Can you work these out from the model? Positions are in its coordinate system, mm. A direction names the side the tool comes from. Round coordinates to 2 decimals unless told otherwise and drop trailing zeros. Order: outer loops, then holes, each group sorted by start corner. A loop starts at its lowest first (then second) coordinate and runs counter-clockwise, first axis right, second up. Notation, with made-up numbers: (-1, -25.5) -> (56, -25.5) arc R20 ccw to (56, 1.5) -> close; hole circle Ø8 at (80, 74.5). An arc over 180 degrees is marked (long way). Use a Markdown table: item, result. Add a question column.
Q1. For faces 5 (the face through (-104.944, -2.465, 3.44)), 6 (the face through (-2.5, -2, -60)), which set-ups out of +Z, -Z, +X, -X, +Y, -Y let a thin tool reach every point of the face, with its end or its side?
Q2. I'm going to push flat-ended pins straight in: pin 1 Ø1.5 at (y, z) = (-3.5, -79.5) entering from -X; pin 2 Ø2 at (x, y) = (-24, -3) entering from -Z; pin 3 Ø3 at (x, y) = (-54.5, -3.5) entering from -Z. Where does each tip first touch, or does it pass through?
Q3. We'd pull the mould along Z, two halves only. Please class faces 1 (the face through (-9.91, -2.46, -93.98)), 2 (the face through (83.17, -2.46, -44.87)), 3 (the face through (86.34, -2.46, 38.41)), 4 (the face through (2.5, -2, -64)): +Z half, -Z half, draft (parallel to the pull), parting line (faces both ways), or undercut.
Q4. I need wall thicknesses on line 1 along X through (y, z) = (-0.45, 17.5); line 2 along Z through (x, y) = (-35, -4.15); line 3 along Z through (x, y) = (-22.5, -3.2). Which ranges of each line are inside material? Lowest first, please. Write a range as [from, to].
Q5. If we section it at B-B on x = 74: List the corners of the cut face in (y, z) for me.
Q6. If we section it at A-A on z = 80: List the corners of the cut face in (x, y) for me, plus the area to 3 significant figures.
Q7. If we section it at C-C on x = -33: List the corners of the cut face in (y, z) for me, plus the area to 3 significant figures.
Q8. If we section it at D-D on x = -69.5: List the corners of the cut face in (y, z) for me.
```python
from build123d import *

# Parameters (mm, degrees)
EXTRUDE_1_DEPTH = 5
EXTRUDE_2_DEPTH = 5
FILLET_1_R      = 2


with BuildPart() as part:
    # 草圖1 → 填料-伸長1 (new body)
    with BuildSketch(Plane(origin=(0, 0, 0), x_dir=(1, 0, 0), z_dir=(0, 1, 0))):
        with BuildLine():
            Line((50.565945697, -26.307511014), (22.900635095, -10.334936491))
            Line((22.900635095, -10.334936491), (20.400635095, -14.665063509))
            Line((20.400635095, -14.665063509), (48.065945697, -30.637638033))
            ThreePointArc((48.065945697, -30.637638033), (30.4, -48.216594654), (6.922542226, -56.578073572))
            Line((6.922542226, -56.578073572), (4.437329437, -24.729741355))
            Line((4.437329437, -24.729741355), (-0.547516958, -25.118722602))
            Line((-0.547516958, -25.118722602), (1.93769583, -56.96705482))
            ThreePointArc((1.93769583, -56.96705482), (-26.556795854, -50.435469602), (-48.065945697, -30.637638033))
            Line((-48.065945697, -30.637638033), (-20.400635095, -14.665063509))
            Line((-20.400635095, -14.665063509), (-22.900635095, -10.334936491))
            Line((-22.900635095, -10.334936491), (-50.565945697, -26.307511014))
            ThreePointArc((-50.565945697, -26.307511014), (-56.956795854, -2.218874948), (-52.459320124, 22.29393936))
            Line((-52.459320124, 22.29393936), (-23.635248961, 8.522030659))
            Line((-23.635248961, 8.522030659), (-21.479693405, 13.033524896))
            Line((-21.479693405, 13.033524896), (-50.303764568, 26.805433596))
            ThreePointArc((-50.303764568, 26.805433596), (-30.4, 48.216594654), (-2.5, 56.945149047))
            Line((-2.5, 56.945149047), (-2.5, 25))
            Line((-2.5, 25), (2.5, 25))
            Line((2.5, 25), (2.5, 56.945149047))
            ThreePointArc((2.5, 56.945149047), (26.556795854, 50.435469602), (45.536777898, 34.284134212))
            Line((45.536777898, 34.284134212), (19.197919523, 16.207710695))
            Line((19.197919523, 16.207710695), (22.027210363, 12.085197706))
            Line((22.027210363, 12.085197706), (48.366068738, 30.161621224))
            ThreePointArc((48.366068738, 30.161621224), (56.956795854, 2.218874948), (50.565945697, -26.307511014))
        make_face()
    extrude(amount=-EXTRUDE_1_DEPTH)

    # 草圖4 → 填料-伸長2 (add)
    with BuildSketch(Plane(origin=(0, 0, 0), x_dir=(1, 0, 0), z_dir=(0, 1, 0))):
        with BuildLine():
            ThreePointArc((48.065945697, -30.637638033), (30.4, -48.216594654), (6.922542226, -56.578073572))
            Line((6.922542226, -56.578073572), (10.658713711, -104.457607775))
            ThreePointArc((10.658713711, -104.457607775), (56, -88.820042783), (89.656889178, -54.650180448))
            Line((89.656889178, -54.650180448), (48.065945697, -30.637638033))
        make_face()
        with BuildLine():
            Line((4.85674931, -94.375113172), (1.93769583, -56.96705482))
            ThreePointArc((1.93769583, -56.96705482), (-12.735400783, -55.559063769), (-26.556796584, -50.435469218))
            ThreePointArc((-26.556796584, -50.435469218), (-9.497439871, -68.99258523), (-8.040249963, -94.157338432))
            ThreePointArc((-8.040249963, -94.157338432), (-1.595470326, -94.486530651), (4.85674931, -94.375113172))
        make_face()
        with BuildLine():
            ThreePointArc((56.956795794, 2.218876491), (55.621252058, -12.460991916), (50.565945697, -26.307511014))
            Line((50.565945697, -26.307511014), (83.060757239, -45.068399205))
            ThreePointArc((83.060757239, -45.068399205), (85.942912679, -39.294602178), (88.424299029, -33.337566517))
            ThreePointArc((88.424299029, -33.337566517), (66.346381744, -21.173940759), (56.956795794, 2.218876491))
        make_face()
        with BuildLine():
            ThreePointArc((-73.083329018, -59.908906012), (-51.510362628, -46.870681896), (-26.556796584, -50.435469218))
            ThreePointArc((-26.556796584, -50.435469218), (-38.602162456, -41.938920512), (-48.065945697, -30.637638033))
            Line((-48.065945697, -30.637638033), (-80.560757239, -49.398526224))
            ThreePointArc((-80.560757239, -49.398526224), (-77.001580057, -54.781444566), (-73.083329018, -59.908906012))
        make_face()
        with BuildLine():
            ThreePointArc((48.366068738, 30.161621224), (54.483260678, 16.750352411), (56.956795794, 2.218876491))
            ThreePointArc((56.956795794, 2.218876491), (64.498052131, 26.271269361), (85.562772016, 40.115608495))
            ThreePointArc((85.562772016, 40.115608495), (82.625471022, 45.861547492), (79.302870836, 51.393624868))
            Line((79.302870836, 51.393624868), (48.366068738, 30.161621224))
        make_face()
        with BuildLine():
            Line((-92.156889178, -50.320053429), (-50.565945697, -26.307511014))
            ThreePointArc((-50.565945697, -26.307511014), (-56.956795854, -2.218874948), (-52.459320124, 22.29393936))
            Line((-52.459320124, 22.29393936), (-95.792298807, 42.998087042))
            ThreePointArc((-95.792298807, 42.998087042), (-104.920413415, -4.08740122), (-92.156889178, -50.320053429))
        make_face()
        with BuildLine():
            ThreePointArc((2.5, 56.945149047), (26.556795854, 50.435469602), (45.536777898, 34.284134212))
            Line((45.536777898, 34.284134212), (85.133585096, 61.459520733))
            ThreePointArc((85.133585096, 61.459520733), (48.920413415, 92.907444004), (2.5, 104.970233876))
            Line((2.5, 104.970233876), (2.5, 56.945149047))
        make_face()
        with BuildLine():
            Line((-84.159620147, 42.981488303), (-50.303764568, 26.805433596))
            ThreePointArc((-50.303764568, 26.805433596), (-41.747859976, 38.808712777), (-30.399998639, 48.216595512))
            ThreePointArc((-30.399998639, 48.216595512), (-55.000611157, 42.721316766), (-77.522522053, 54.041729936))
            ThreePointArc((-77.522522053, 54.041729936), (-81.030000696, 48.624983159), (-84.159620147, 42.981488303))
        make_face()
        with BuildLine():
            ThreePointArc((-30.399998639, 48.216595512), (-17.019088969, 54.399913701), (-2.5, 56.945149047))
            Line((-2.5, 56.945149047), (-2.5, 94.466925429))
            ThreePointArc((-2.5, 94.466925429), (-8.941332621, 94.076046744), (-15.34097001, 93.246472529))
            ThreePointArc((-15.34097001, 93.246472529), (-14.836019776, 68.044623914), (-30.399998639, 48.216595512))
        make_face()
    extrude(amount=-EXTRUDE_2_DEPTH)

    # 圓角1
    fillet_1_edges = [part.edges().sort_by_distance(p)[0] for p in [
        (-80.560757239, -2.5, 49.398526224),
        (4.85674931, -2.5, 94.375113172),
        (-84.159620147, -2.5, -42.981488303),
        (-2.5, -2.5, -94.466925429),
        (79.302870836, -2.5, -51.393624868),
        (83.060757239, -2.5, 45.068399205),
        (4.437329437, -2.5, 24.729741355),
        (-0.547516958, -2.5, 25.118722602),
        (-20.400635095, -2.5, 14.665063509),
        (-22.900635095, -2.5, 10.334936491),
        (-23.635248961, -2.5, -8.522030659),
        (-21.479693405, -2.5, -13.033524896),
        (-2.5, -2.5, -25),
        (2.5, -2.5, -25),
        (19.197919523, -2.5, -16.207710695),
        (22.027210363, -2.5, -12.085197706),
        (22.900635095, -2.5, 10.334936491),
        (20.400635095, -2.5, 14.665063509),
        (-95.792298807, -2.5, -42.998087042),
        (-92.156889178, -2.5, 50.320053429),
        (10.658713711, -2.5, 104.457607775),
        (89.656889178, -2.5, 54.650180448),
        (85.133585096, -2.5, -61.459520733),
        (2.5, -2.5, -104.970233876),
    ]]
    fillet(fillet_1_edges, radius=FILLET_1_R)


solid = part.part
```
Answer below:
| question | item | result |
|---|---|---|
| 1 | face 5 | -X, +Y, -Y |
| 1 | face 6 | -Z, +Y, -Y |
| 2 | pin 1 | x = -12.92 |
| 2 | pin 2 | z = -54.34 |
| 2 | pin 3 | z = -42.86 |
| 3 | face 1 | -Z half |
| 3 | face 2 | undercut |
| 3 | face 3 | undercut |
| 3 | face 4 | draft |
| 4 | line 1 | [-103.53, -35.31], [-25.31, 25.31], [35.31, 63.48] |
| 4 | line 2 | [-45.75, -19.49], [-13.95, 17.32], [23.09, 47.22] |
| 4 | line 3 | [-54.88, -13.23], [-10.9, 11.42], [15.88, 52.91] |
| 5 | outline | (-5, -74.49) -> (0, -74.49) -> (0, -53.82) -> (-5, -53.82) -> close; (-5, -47.75) -> (0, -47.75) -> (0, -35.13) -> (-5, -35.13) -> close; (-5, 27.77) -> (0, 27.77) -> (0, 39.84) -> (-5, 39.84) -> close; (-5, 45.61) -> (0, 45.61) -> (0, 74.49) -> (-5, 74.49) -> close |
| 6 | outline | (-6.7, -5) -> (3.74, -5) -> (3.74, 0) -> (-6.7, 0) -> close; (8.75, -5) -> (68.01, -5) -> (68.01, 0) -> (8.75, 0) -> close |
| 6 | area | 348 mm² |
| 7 | outline | (-5, -46.72) -> (0, -46.72) -> (0, -18.54) -> (-5, -18.54) -> close; (-5, -13) -> (0, -13) -> (0, 16.17) -> (-5, 16.17) -> close; (-5, 21.94) -> (0, 21.94) -> (0, 47.78) -> (-5, 47.78) -> close |
| 7 | area | 416 mm² |
| 8 | outline | (-5, -47.67) -> (0, -47.67) -> (0, -35.98) -> (-5, -35.98) -> close; (-5, -30.44) -> (0, -30.44) -> (0, 37.24) -> (-5, 37.24) -> close; (-5, 43.01) -> (0, 43.01) -> (0, 56.09) -> (-5, 56.09) -> close |
